from build123d import *

# Parameters (mm, degrees)
F1_DEPTH = 300
F2_T     = -2.5


with BuildPart() as f1:
    # F0 (on Top) → F1 (new body)
    with BuildSketch(Plane.XY):
        with BuildLine():
            ThreePointArc((-158.7704400152, 367.1402284923), (-176.7766952966, 176.7766952966), (-367.1402284923, 158.7704400152))
            ThreePointArc((-367.1402284923, 158.7704400152), (-369.5518130045, 153.073372946), (-371.875, 147.3396904266))
            ThreePointArc((-371.875, 147.3396904266), (-550, 0), (-371.875, -147.3396904266))
            ThreePointArc((-371.875, -147.3396904266), (-369.5518130045, -153.073372946), (-367.1402284923, -158.7704400152))
            ThreePointArc((-367.1402284923, -158.7704400152), (-176.7766952966, -176.7766952966), (-158.7704400152, -367.1402284923))
            ThreePointArc((-158.7704400152, -367.1402284923), (-153.073372946, -369.5518130045), (-147.3396904266, -371.875))
            ThreePointArc((-147.3396904266, -371.875), (0, -550), (147.3396904266, -371.875))
            ThreePointArc((147.3396904266, -371.875), (153.073372946, -369.5518130045), (158.7704400152, -367.1402284923))
            ThreePointArc((158.7704400152, -367.1402284923), (176.7766952966, -176.7766952966), (367.1402284923, -158.7704400152))
            ThreePointArc((367.1402284923, -158.7704400152), (369.5518130045, -153.073372946), (371.875, -147.3396904266))
            ThreePointArc((371.875, -147.3396904266), (550, 0), (371.875, 147.3396904266))
            ThreePointArc((371.875, 147.3396904266), (369.5518130045, 153.073372946), (367.1402284923, 158.7704400152))
            ThreePointArc((367.1402284923, 158.7704400152), (176.7766952966, 176.7766952966), (158.7704400152, 367.1402284923))
            ThreePointArc((158.7704400152, 367.1402284923), (153.073372946, 369.5518130045), (147.3396904266, 371.875))
            ThreePointArc((147.3396904266, 371.875), (0, 550), (-147.3396904266, 371.875))
            ThreePointArc((-147.3396904266, 371.875), (-153.073372946, 369.5518130045), (-158.7704400152, 367.1402284923))
        make_face()
    extrude(amount=F1_DEPTH)

    # F2
    f2_openings = [f1.faces().sort_by_distance(p)[0] for p in [
        (0, 0, 300),
    ]]
    offset(amount=F2_T, openings=f2_openings, kind=Kind.INTERSECTION)


solid = f1.part
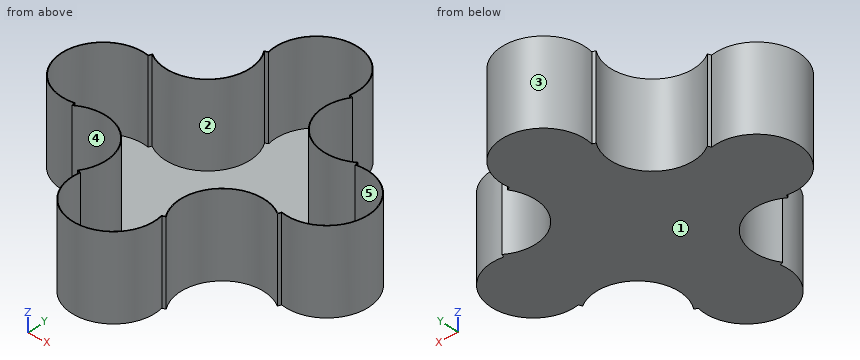
For this review, take the finished solid that the model builds, in its own axes (mm). Face numbers are marked on the shaded views. A direction names the side the tool comes from. Give positions to 0.01 mm unless a question says otherwise; leave off trailing zeros. Loops run counter-clockwise (first coordinate to the right, second up) from the corner with the lowest first, then second, coordinate; pieces in that order, holes last.
Item 1: Insertion check: pin 1 (1 mm diameter, centred on y = -67.5, z = 77, fed in from +X); pin 2 (12 mm diameter, centred on y = -235.5, z = 115.5, fed in from +X); pin 3 (8 mm diameter, centred on y = 333, z = 225, fed in from -X). Each pin has a flat end and moves straight along its axis. Give the tip position at first contact, or say it passes through.
Item 2: Tool access review of the marked faces 4 and 5: name each direction out of +Z, -Z, +X, -X, +Y, -Y from which nothing blocks a thin tool from reaching the whole face with its end or side.
Item 3: Take a section at A-A, the plane y = 400. State the section outline as (x, z) points.
Item 4: Draft analysis for pull direction X (two halves, no side actions). For the marked faces 1, 2 and 3, state which applies: +X half, -X half, draft (parallel to the pull), parting line (faces both ways), or undercut.
Item 5: For line 1 along Y through (x, z) = (-151, 131); line 2 along X through (y, z) = (-409, 262.5); line 3 along X through (y, z) = (400, 166.5), list the stretches that pass through material, from the lowest coordinate up.
Calculated:
1. pin 1: stops at x = 534.21
1. pin 2: stops at x = 142.65
1. pin 3: stops at x = -142.96
2. face 4: +Z, -Z
2. face 5: +Z
3. outline: (-150, 0) - (150, 0) - (150, 300) - (147.5, 300) - (147.5, 2.5) - (-147.5, 2.5) - (-147.5, 300) - (-150, 300) - close
4. face 1: draft
4. face 2: undercut
4. face 3: parting line
5. line 1: y = -370.4 to -367.7, -359.48 to -354.38, -211.31 to -206.2, 206.2 to 211.31, 354.38 to 359.48, 367.7 to 370.4
5. line 2: x = -149.73 to -147.23, 147.23 to 149.73
5. line 3: x = -150 to -147.5, 147.5 to 150
